Autodesk Inventor part; units mm, degrees
ref_plane "Work Plane1" through (19.2904, 0, 0) normal (0.342, 0, -0.9397) x (0, 1, 0)
ref_plane "YZ Plane" through (0, 0, 0) normal (1, 0, 0) x (0, 1, 0)
ref_plane "XZ Plane" through (0, 0, 0) normal (0, 1, 0) x (-1, 0, 0)
sketch "Sketch1" plane through (0, 0, 0) normal (0, 0, 1) x (1, 0, 0)
  circle A0 centre (0, 0) radius 85
  dimension "d0" = 170
extrude "Extrusion1" add sketch "Sketch1" along normal blind 8
sketch "Sketch2" plane through (0, 0, 8) normal (0, 0, 1) x (1, 0, 0)
  circle A0 centre (0, 0) radius 71.75
  dimension "d3" = 143.5
extrude "Extrusion2" add sketch "Sketch2" along normal blind 2
sketch "Sketch3" plane through (0, 0, 10) normal (0, 0, 1) x (1, 0, 0)
  circle A0 centre (0, 0) radius 6.5
  dimension "d6" = 13
extrude "Extrusion3" cut sketch "Sketch3" against normal through all
sketch "Sketch4" plane through (0, 0, 0) normal (0, 1, 0) x (-1, 0, 0)
  line L0 (0, 53) -> (-39.9771, -56.8361) construction
  line L1 (85, 8) -> (-85, 8) construction
  line L2 (0, -78.8034) -> (0, 74.9672) construction
  point P0 (0, 0)
  dimension "d9" = 45
  dimension "d10" = 20
ref_plane "Work Plane1" through (19.2904, 0, 0) normal (0.342, 0, -0.9397) x (0, 1, 0)
sketch "Sketch5" plane through (19.2904, 0, 0) normal (0.342, 0, -0.9397) x (0, 1, 0)
  line L0 (0, 0) -> (0, -2.8191) construction
  line L1 (-5, 0) -> (-5, -2.8191)
  line L2 (5, -2.8191) -> (5, 0)
  arc A0 (5, 0) -> (-5, 0) centre (0, 0) ccw
  arc A1 (-5, -2.8191) -> (5, -2.8191) centre (0, -2.8191) ccw
  line L3 (0, 0) -> (0, -2) construction
  line L4 (-5, 0) -> (-5, -2)
  line L5 (5, -2) -> (5, 0)
  arc A2 (5, 0) -> (-5, 0) centre (0, 0) ccw
  arc A3 (-5, -2) -> (5, -2) centre (0, -2) ccw
  point P0 (0, -18.1271)
  point P1 (0, -1.4095)
  point P2 (0, -1)
  point P3 (-5, -2)
  point P4 (5, -2)
  dimension "d12" = 10
  dimension "d13" = 2.8191
  dimension "d37" = 2
extrude "Extrusion4" cut sketch "Sketch5" against normal through all both and the other way through all
sketch "Sketch10" plane through (0, 0, 0) normal (0, 0, -1) x (-1, 0, 0)
  line L0 (119, 0) -> (-119, 0)
  line L1 (0, 0) -> (-18.2904, -11.65) construction
  line L2 (-18.2904, -11.65) -> (-18.2904, -5) construction
  line L3 (-16.2904, -5) -> (-19.2904, -5) construction
  point P0 (-18.2904, 11.65)
  point P1 (-30, 0)
  dimension "d50" = 30
  dimension "d60" = 11.65
  dimension "d61" = 1
hole "Hole1" at (18.2904, -11.65, 0) at (18.2904, 11.65, 0) at (30, 0, 0) direction (0, 0, 1) diameter 2.459 depth 6 tip angle 118
sketch "Sketch12" plane through (0, 0, 0) normal (1, 0, 0) x (0, 1, 0)
  line L0 (85, 8) -> (-85, 8)
  circle A0 centre (-76, 8) radius 2
  line L1 (0, -78.8034) -> (0, 74.9672)
  point P0 (0, 0)
  dimension "d63" = 4
  dimension "d64" = 76
revolve "Revolution1" cut sketch "Sketch12" angle 360 about axis through (0, 0, -10) along (0, 0, 1)
properties part number "Deckel" material "Polycarbonate, Clear"
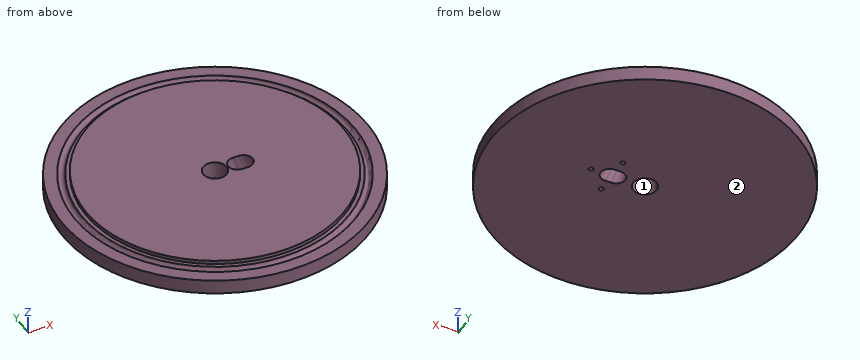
The listing builds one solid part. Answer for the finished solid, in the listing's coordinates (mm). Face numbers are marked on the shaded views. Coordinates: 2 decimals unless noted, no trailing zeros. Order: outer loops, then holes, each group sorted by start corner. A loop starts at its lowest first (then second) coordinate and runs counter-clockwise, first axis right, second up. Notation, with made-up numbers: (83, 31) -> (116, 31) arc R21 cw to (116, 51) -> close; hole circle Ø4 at (-11.75, 74.25). An arc over 180 degrees is marked (long way). Answer in a Markdown table with one row per item. Add a question column.
Item 1: Each of these flat-tipped pins is pushed along its axis until it touches: P1, Ø11.5, axis at x = 0, y = 0, coming from the +Z side; P2, Ø3, axis at x = -32.5, z = 2.5, coming from the -Y side; P3, Ø5.5, axis at x = 16, z = 6, coming from the +Y side; P4, Ø2, axis at x = 18.29, y = -11.65, coming from the -Z side. Where does it stop, or does it pass through?
Item 2: Determine the mould class of the marked faces 1 and 2 for opening direction Y: +Y half, -Y half, draft (parallel to the pull), parting line (faces both ways), or undercut.
Item 3: Find section A-A (x = 0). Write down the section's boundary in (y, z), then the cut area to 3 significant figures.
Item 4: Find the intervals of material crossed by L1, parallel to Y at x = 53, z = 7.5; L2, parallel to Y at x = 30, z = 2.6; L3, parallel to Z at x = 56, y = -63, in increasing order. Write a range as from..to.
Item 5: Find section B-B (z = 3.25). State how many separate pieces and enclosed holes the cut face has, then the cut area to 3 significant figures.
Result set:
| question | item | result |
|---|---|---|
| 1 | P1 | passes through |
| 1 | P2 | stops at y = -79.15 |
| 1 | P3 | stops at y = 83.96 |
| 1 | P4 | stops at z = 6.14 |
| 2 | face 1 | undercut |
| 2 | face 2 | draft |
| 3 | outline | (-85, 0) -> (-6.5, 0) -> (-6.5, 10) -> (-71.75, 10) -> (-71.75, 8) -> (-74, 8) arc R2 cw to (-78, 8) -> (-85, 8) -> close; (6.5, 0) -> (85, 0) -> (85, 8) -> (78, 8) arc R2 cw to (74, 8) -> (71.75, 8) -> (71.75, 10) -> (6.5, 10) -> close |
| 3 | area | 1,500 mm² |
| 4 | L1 | y = -66.45..-57.14, -51.73..51.73, 57.14..66.45 |
| 4 | L2 | y = -79.53..-1.23, 1.23..79.53 |
| 4 | L3 | z = 0..8 |
| 5 | separate pieces | 1 |
| 5 | enclosed holes | 5 |
| 5 | area | 22,400 mm² |
